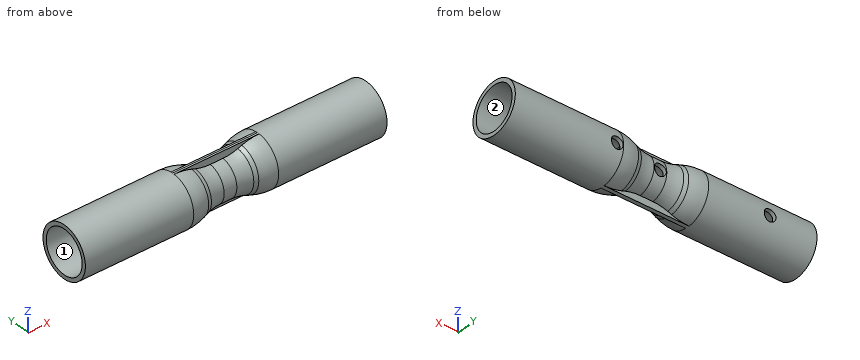
Autodesk Inventor part; units mm, degrees
ref_plane "YZ Plane" through (0, 0, 0) normal (1, 0, 0) x (0, 1, 0)
ref_plane "XZ Plane" through (0, 0, 0) normal (0, 1, 0) x (-1, 0, 0)
ref_plane "XY Plane" through (0, 0, 0) normal (0, 0, 1) x (1, 0, 0)
sketch "Sketch1" plane through (0, 0, 0) normal (0, 0, 1) x (1, 0, 0)
  line L0 (0, 0) -> (70, 0)
  line L1 (23.4899, 8.9035) -> (21.5101, 9.5965)
  line L2 (46.5101, 8.9035) -> (48.4899, 9.5965)
  arc A0 (21.5101, 9.5965) -> (13.2514, 11) centre (13.2514, -14) ccw
  arc A1 (23.4899, 8.9035) -> (31.7486, 7.5) centre (31.7486, 32.5) ccw
  arc A2 (38.2514, 7.5) -> (46.5101, 8.9035) centre (38.2514, 32.5) ccw
  arc A3 (56.7486, 11) -> (48.4899, 9.5965) centre (56.7486, -14) ccw
  arc A4 (22.1708, 11.4842) -> (13.2514, 13) centre (13.2514, -14) ccw
  line L3 (22.1708, 11.4842) -> (24.1506, 10.7913)
  arc A5 (24.1506, 10.7913) -> (31.7486, 9.5) centre (31.7486, 32.5) ccw
  arc A6 (38.2514, 9.5) -> (45.8494, 10.7913) centre (38.2514, 32.5) ccw
  line L4 (45.8494, 10.7913) -> (47.8292, 11.4842)
  arc A7 (56.7486, 13) -> (47.8292, 11.4842) centre (56.7486, -14) ccw
  line L5 (31.7486, 9.5) -> (38.2514, 9.5)
  line L6 (31.7486, 7.5) -> (38.2514, 7.5)
  line L7 (-42.25, 13) -> (-42.25, 11)
  line L8 (112.25, 13) -> (112.25, 11)
  line L9 (56.7486, 13) -> (112.25, 13)
  line L10 (56.7486, 11) -> (112.25, 11)
  line L11 (13.2514, 13) -> (-42.25, 13)
  line L12 (13.2514, 11) -> (-42.25, 11)
  point P0 (17.5, 11)
  point P1 (52.5, 11)
  point P2 (42.5, 7.5)
  point P3 (27.5, 7.5)
  dimension "d8" = 25
  dimension "d43" = 154.5
revolve "Revolution1" add sketch "Sketch1" angle 360 about axis through (0, 0, 0) along (1, 0, 0)
sketch "Sketch3" plane through (0, 0, 0) normal (0, 1, 0) x (-1, 0, 0)
  circle A0 centre (-35, 0) radius 3
  line L0 (-70, 11) -> (-70, -11)
  line L1 (-56.7486, 11) -> (-56.7486, -11)
  line L2 (-70, 0) -> (-60, 0)
  circle A1 centre (-60, 0) radius 3
  line L3 (-13.2514, 11) -> (-13.2514, -11)
  circle A2 centre (18.2486, 0) radius 3
  dimension "d12" = 6
  dimension "d13" = 10
  dimension "d14" = 6
  dimension "d51" = 6
extrude "Extrusion1" cut sketch "Sketch3" along normal blind 20
sketch "Sketch4" plane through (0, 0, 0) normal (0, 1, 0) x (-1, 0, 0)
  line L0 (-56.7486, -13) -> (-13.2514, -13)
  arc A0 (-56.7486, -12) -> (-48.1595, -10.5403) centre (-56.7486, 14) ccw
  line L1 (-48.1595, -10.5403) -> (-46.1798, -9.8474)
  arc A1 (-38.2514, -8.5) -> (-46.1798, -9.8474) centre (-38.2514, -32.5) ccw
  line L2 (-31.7486, -8.5) -> (-38.2514, -8.5)
  arc A2 (-23.8202, -9.8474) -> (-31.7486, -8.5) centre (-31.7486, -32.5) ccw
  line L3 (-23.8202, -9.8474) -> (-21.8405, -10.5403)
  arc A3 (-21.8405, -10.5403) -> (-13.2514, -12) centre (-13.2514, 14) ccw
  line L4 (-56.7486, -13) -> (-56.7486, -12)
  line L5 (-13.2514, -12) -> (-13.2514, -13)
  point P0 (0, 0)
  point P1 (-22.1708, -11.4842)
  point P2 (-38.2514, -9.5)
  point P3 (-45.8494, -10.7913)
  point P4 (-47.8292, -11.4842)
  point P5 (-38.2514, -8.5)
  point P6 (-48.1595, -10.5403)
extrude "Extrusion3" add sketch "Sketch4" along normal mid plane 2
mirror "Mirror1" about plane through (0, 0, 0) normal (0, 0, 1) of "Extrusion3"
sketch "Sketch6" plane through (-42.25, 0, 0) normal (-1, 0, 0) x (0, 0, 1)
  line L0 (13, 1) -> (13, 0)
  circle A0 centre (0, 0) radius 13
  circle A1 centre (0, 0) radius 15
  dimension "d46" = 30
extrude "Extrusion6" cut sketch "Sketch6" against normal up to surface (154.5 mm away)
properties part number "Venturi Valve"
Can you work these out from the model? Positions are in its coordinate system, mm. Face numbers are marked on the shaded views. A direction names the side the tool comes from. Coordinates: 2 decimals unless noted, no trailing zeros. Loops run counter-clockwise (first coordinate to the right, second up) from the corner with the lowest first, then second, coordinate; pieces in that order, holes last. Notation, with made-up numbers: M 22,36 L 38,36 A19 ccw 38,57 Z; hole C 14,3 d7. An arc over 180 degrees is marked long. Put each result on its own line as item: value. Start each with the question number.
(1) I need wall thicknesses on probe 1 along Z at (x, y) = (-13.5, 0); probe 2 along Y at (x, z) = (32.5, -9.5); probe 3 along Y at (x, z) = (-27.5, 9.75). Which ranges of each line are inside material? Lowest first, please.
(2) Which directions (+Z, -Z, +X, -X, +Y, -Y) give clear straight access to the entire face, cutting with the end or side of a thin tool? Please do the marked faces 1 and 2.
(3) Imagine slicing it at C-C on x = 35. List the corners of the cut face in (y, z) for me, and give its area (3 significant figures).
(4) Imagine slicing it at B-B on x = 69.5. List the corners of the cut face in (y, z) for me.
(5) Will these pins go through, and if not, where does the flat tip stop? pin 1 Ø1.8 at (x, z) = (34, -10.5) entering from +Y; pin 2 Ø3 at (x, y) = (66, 3.5) entering from +Z; pin 3 Ø4 at (x, z) = (41.5, 10.5) entering from -Y.
(6) Imagine slicing it at A-A on z = 0. Give the number of separate pieces and of enclosed holes in the cut face, and give its area (3 significant figures).
Worked answers:
1. probe 1: z = -13 to -11, 11 to 13
1. probe 2: y = -1 to 1
1. probe 3: y = -8.6 to -5.09, 5.09 to 8.6
2. face 1: -X
2. face 2: +X
3. outline: M -1,-12.96 A13 ccw 1,-12.96 L 1,-9.45 A9.5 ccw 9.01,-3 L 6.87,-3 A7.5 cw long 6.87,3 L 9.01,3 A9.5 ccw 1,9.45 L 1,12.96 A13 ccw -1,12.96 L -1,9.45 A9.5 ccw -1,-9.45 Z
3. area: 109 mm2
4. outline: C 0,0 d26; hole C 0,0 d22
5. pin 1: stops at y = 1
5. pin 2: stops at z = 12.85
5. pin 3: stops at y = -4.79
6. separate pieces: 5
6. enclosed holes: 0
6. area: 585 mm2
